Geometry check sheet. Reference: the model listing, model coordinates, mm. A direction names the side the tool comes from. Round coordinates to 2 decimals unless told otherwise and drop trailing zeros. Order: outer loops, then holes, each group sorted by start corner. A loop starts at its lowest first (then second) coordinate and runs counter-clockwise, first axis right, second up.
(1) Release check for a two-part mould opening along Y. For faces 5 (the face through (25.1, 12.89, 0.96)), 6 (the face through (0, -8, 3)), 7 (the face through (-2, -11, -2)), 8 (the face through (17, -13.75, 1)) record: +Y half, -Y half, draft (parallel to the pull), parting line (faces both ways), or undercut.
(2) Material ranges on line 1 along Y through (x, z) = (-1.5, 2); line 2 along X through (y, z) = (-2, 0.9); line 3 along Y through (x, z) = (11, -1.4), recorded low to high.
(3) Sectioned sample at A-A (y = 0). Record the boundary of the cut face in (x, z), plus the area to 3 significant figures.
(4) Sectioned sample at C-C (x = -12.75). Record the boundary of the cut face in (y, z).
(5) Set-up check for faces 1 (the face through (-10, -16, 1)), 2 (the face through (0, 4.75, 1)), 3 (the face through (9.55, -15.78, 3.57)), 4 (the face through (10, -16, 1)): record each of +Z, -Z, +X, -X, +Y, -Y from which the full face is reachable in a straight line by a thin tool's end or side.
(6) Sectioned sample at D-D (x = -22). Record the boundary of the cut face in (y, z).
(7) Go/stop test with flat-tipped pins: pin 1 (11 mm diameter, centred on x = 7, y = 0, fed in from -Z); pin 2 (1 mm diameter, centred on x = -16, z = -1, fed in from -Y); pin 3 (1.8 mm diameter, centred on x = 0.5, y = -8.5, fed in from -Z). Record where each tip stops, or that it passes through.
(8) Sectioned sample at B-B (z = 1.6). Record the boundary of the cut face in (x, y).
from build123d import *

# Parameters (mm, degrees)
SKETCH_1_W          = 52
SKETCH_1_H          = 27.5
SKETCH_1_R          = 8.25
EXTRUDE_1_DEPTH     = 4
SKETCH_1_3_W        = 52
SKETCH_1_3_H        = 27.5
SKETCH_1_3_W_2      = 46
SKETCH_1_3_H_2      = 21.5
EXTRUDE_2_DEPTH     = 2
CUT_EXTRUDE_1_DEPTH = 3
FILLET_1_R          = 3
SKETCH_2_W          = 20
SKETCH_2_H          = 6
EXTRUDE_3_DEPTH     = 4
FILLET_2_R          = 1.5


with BuildPart() as part:
    # Sketch 1 → Extrude 1 (new body)
    with BuildSketch(Plane.XY):
        Rectangle(SKETCH_1_W, SKETCH_1_H)
        with Locations((-12.75, 0)):
            Circle(SKETCH_1_R, mode=Mode.SUBTRACT)
        with Locations((12.75, 0)):
            Circle(SKETCH_1_R, mode=Mode.SUBTRACT)
    extrude(amount=EXTRUDE_1_DEPTH)

    # Sketch 1_3 → Extrude 2 (add)
    with BuildSketch(Plane.XY):
        Rectangle(SKETCH_1_3_W, SKETCH_1_3_H)
        Rectangle(SKETCH_1_3_W_2, SKETCH_1_3_H_2, mode=Mode.SUBTRACT)
    extrude(amount=-EXTRUDE_2_DEPTH)

    # Sketch 1_4 → Cut-Extrude 1 (cut)
    with BuildSketch(Plane.XY):
        with BuildLine():
            Line((5.5, 10.75), (-5.5, 10.75))
            Line((-5.5, 10.75), (-5.5, 5.75))
            ThreePointArc((-5.5, 5.75), (-5.207106781, 5.042893219), (-4.5, 4.75))
            Line((-4.5, 4.75), (4.5, 4.75))
            ThreePointArc((4.5, 4.75), (5.207106781, 5.042893219), (5.5, 5.75))
            Line((5.5, 5.75), (5.5, 10.75))
        make_face()
        with BuildLine():
            Line((-5.5, -5.75), (-5.5, -10.75))
            Line((-5.5, -10.75), (5.5, -10.75))
            Line((5.5, -10.75), (5.5, -5.75))
            ThreePointArc((5.5, -5.75), (5.207106781, -5.042893219), (4.5, -4.75))
            Line((4.5, -4.75), (-4.5, -4.75))
            ThreePointArc((-4.5, -4.75), (-5.207106781, -5.042893219), (-5.5, -5.75))
        make_face()
    extrude(amount=CUT_EXTRUDE_1_DEPTH, mode=Mode.SUBTRACT)

    # Fillet 1
    fillet_1_edges = [part.edges().sort_by_distance(p)[0] for p in [
        (-26, 13.75, 1),
        (26, 13.75, 1),
    ]]
    fillet(fillet_1_edges, radius=FILLET_1_R)

    # Sketch 2 → Extrude 3 (add)
    with BuildSketch(Plane.XZ.offset(13.75)):
        with Locations((0, 1)):
            Rectangle(SKETCH_2_W, SKETCH_2_H)
    extrude(amount=EXTRUDE_3_DEPTH)

    # Fillet 2
    fillet_2_edges = [part.edges().sort_by_distance(p)[0] for p in [
        (-10, -15.75, -2),
        (-10, -15.75, 4),
        (10, -15.75, -2),
        (10, -15.75, 4),
    ]]
    fillet(fillet_2_edges, radius=FILLET_2_R)


solid = part.part
Answer below:
1. face 5: +Y half
1. face 6: undercut
1. face 7: draft
1. face 8: -Y half
2. line 1: y = -17.75 to -10.75, -4.75 to 4.75, 10.75 to 13.75
2. line 2: x = -26 to -20.75, -4.75 to 4.75, 20.75 to 26
2. line 3: y = -13.75 to -10.75, 10.75 to 13.75
3. outline: (-26, -2) - (-23, -2) - (-23, 0) - (-21, 0) - (-21, 4) - (-26, 4) - close; (-4.5, 0) - (4.5, 0) - (4.5, 4) - (-4.5, 4) - close; (21, 0) - (23, 0) - (23, -2) - (26, -2) - (26, 4) - (21, 4) - close
3. area: 88.0 mm2
4. outline: (-13.75, -2) - (-10.75, -2) - (-10.75, 0) - (-8.25, 0) - (-8.25, 4) - (-13.75, 4) - close; (8.25, 0) - (10.75, 0) - (10.75, -2) - (13.75, -2) - (13.75, 4) - (8.25, 4) - close
5. face 1: +Z, -Z, -X, -Y
5. face 2: -Z
5. face 3: +Z, +X, -Y
5. face 4: +Z, -Z, +X, -Y
6. outline: (-13.75, -2) - (-10.75, -2) - (-10.75, 0) - (10.75, 0) - (10.75, -2) - (13.75, -2) - (13.75, 4) - (-13.75, 4) - close
7. pin 1: stops at z = 0
7. pin 2: stops at y = -13.75
7. pin 3: stops at z = 3
8. outline: (-26, -13.75) - (-10, -13.75) - (-10, -17.75) - (10, -17.75) - (10, -13.75) - (26, -13.75) - (26, 10.75) arc R3 ccw to (23, 13.75) - (-23, 13.75) arc R3 ccw to (-26, 10.75) - close; hole circle Ø16.5 at (-12.75, 0); hole (-5.5, -10.75) - (5.5, -10.75) - (5.5, -5.75) arc R1 ccw to (4.5, -4.75) - (-4.5, -4.75) arc R1 ccw to (-5.5, -5.75) - close; hole (-5.5, 5.75) arc R1 ccw to (-4.5, 4.75) - (4.5, 4.75) arc R1 ccw to (5.5, 5.75) - (5.5, 10.75) - (-5.5, 10.75) - close; hole circle Ø16.5 at (12.75, 0)
